```python
from build123d import *

# Parameters (mm, degrees)
ESQUISSE1_R        = 1.75
BOSS_EXTRU_1_DEPTH = 0.805


with BuildPart() as part:
    # Esquisse1 → Boss.-Extru.1 (new, symmetric)
    with BuildSketch(Plane(origin=(0, 0, 0), x_dir=(1, 0, 0), z_dir=(0, 1, 0))):
        with BuildLine():
            Line((-60.5, 58), (60.5, 58))
            ThreePointArc((60.5, 58), (64.035533906, 56.535533906), (65.5, 53))
            Line((65.5, 53), (65.5, -53))
            ThreePointArc((65.5, -53), (64.035533906, -56.535533906), (60.5, -58))
            Line((60.5, -58), (-60.5, -58))
            ThreePointArc((-60.5, -58), (-64.035533906, -56.535533906), (-65.5, -53))
            Line((-65.5, -53), (-65.5, 53))
            ThreePointArc((-65.5, 53), (-64.035533906, 56.535533906), (-60.5, 58))
        make_face()
        with Locations(Location((-60, 52.5, 0), (0, 0, 90))):
            Circle(ESQUISSE1_R, mode=Mode.SUBTRACT)
        with Locations(Location((60, 52.5, 0), (0, 0, 90))):
            Circle(ESQUISSE1_R, mode=Mode.SUBTRACT)
        with Locations(Location((60, -52.5, 0), (0, 0, 90))):
            Circle(ESQUISSE1_R, mode=Mode.SUBTRACT)
        with Locations(Location((-60, -52.5, 0), (0, 0, 90))):
            Circle(ESQUISSE1_R, mode=Mode.SUBTRACT)
    extrude(amount=BOSS_EXTRU_1_DEPTH, both=True)


solid = part.part
```
Input: part model. Units: mm. Frame: model coordinates. Round coordinates to 2 decimals unless told otherwise and drop trailing zeros. One line per item, written item: value. Start each with the question number.
(1) Ray query, line 1 (Z direction, x = -60, y = -0.4); line 2 (X direction, y = -0.25, z = -52.5). Return the intervals inside material, ascending. Write a range as [from, to].
(2) Draft query along X for faces 1 (the cylindrical face through (-59.33, -0.011, -54.117)), 2 (the flat face through (1, 0.805, -1)), 3 (the cylindrical face through (64, 0.01, -56.57)). Return one class per face: +X half, -X half, draft (parallel to the pull), parting line (faces both ways), or undercut.
(3) Contact query for a flat-ended pin moving along its axis: P1, Ø4.5, axis at x = -60, z = 52.5, coming from the -Y side (3 decimals). Output: stop coordinate, or through.
Results below:
1. line 1: [-58, -54.25], [-50.75, 50.75], [54.25, 58]
1. line 2: [-65.5, -61.75], [-58.25, 58.25], [61.75, 65.5]
2. face 1: undercut
2. face 2: draft
2. face 3: +X half
3. P1: y = -0.805
